from build123d import *

# Parameters (mm, degrees)
SKETCH_1_W               = 17
SKETCH_1_H               = 27
SKETCH_1_R               = 1.5
EXTRUDE_1_DEPTH          = 4
CUT_EXTRUDE_1_DEPTH      = 1
CUT_EXTRUDE_1_DEPTH_BACK = 4
SKETCH_5_W               = 11.75
SKETCH_5_H               = 10
SKETCH_5_R               = 3
EXTRUDE_2_DEPTH          = 4


with BuildPart() as part:
    # Эскиз1 → Бобышка-Вытянуть1 (new body)
    with BuildSketch(Plane.XY):
        with Locations((8.5, 13.5)):
            Rectangle(SKETCH_1_W, SKETCH_1_H)
        with Locations((4, 14.4)):
            Circle(SKETCH_1_R, mode=Mode.SUBTRACT)
        with Locations((4, 4.4)):
            Circle(SKETCH_1_R, mode=Mode.SUBTRACT)
    extrude(amount=EXTRUDE_1_DEPTH)

    # Эскиз2 → Вырез-Вытянуть1 (cut, two sides)
    with BuildSketch(Plane.XY.offset(4)) as cut_extrude_1_sk:
        Polygon((11.25, 5.25), (11.25, 0), (14.25, 0), (14.25, 5.25), (15.5, 5.25), (15.5, 7.75), (14.25, 7.75), (14.25, 13), (11.25, 13), (11.25, 7.75), (10, 7.75), (10, 5.25), align=None)
    extrude(amount=CUT_EXTRUDE_1_DEPTH, mode=Mode.SUBTRACT)
    extrude(cut_extrude_1_sk.sketch, amount=-CUT_EXTRUDE_1_DEPTH_BACK, mode=Mode.SUBTRACT)

    # Эскиз5 → Бобышка-Вытянуть2 (add)
    with BuildSketch(Plane.XY.offset(4)):
        with Locations((-5.875, 22)):
            Rectangle(SKETCH_5_W, SKETCH_5_H)
        with Locations((-6.75, 21.5)):
            Circle(SKETCH_5_R, mode=Mode.SUBTRACT)
    extrude(amount=-EXTRUDE_2_DEPTH)


solid = part.part
The model under review builds one solid part; all positions refer to its coordinate system, in mm. A direction names the side the tool comes from. Round coordinates to 2 decimals unless told otherwise and drop trailing zeros. Loops run counter-clockwise (first coordinate to the right, second up) from the corner with the lowest first, then second, coordinate; pieces in that order, holes last. Notation, with made-up numbers: (80.5, 15.5) -> (88.5, 15.5) arc R32 cw to (88.5, 46.5) -> close; hole circle Ø9 at (-10, 34). An arc over 180 degrees is marked (long way). Answer as CSV lines item,"result".
1) Draft analysis for pull direction Y (two halves, no side actions). For faces 1 (the face through (2, 27, 2)), 2 (the face through (-11.75, 22, 2)), 3 (the face through (-3.98, 20.35, 2.03)), state which applies: pulls with the +Y half, pulls with the -Y half, needs draft (parallel to the pull), parting line crosses it, or undercut.
Geometry results:
face 1,"pulls with the +Y half"
face 2,"needs draft"
face 3,"undercut"
2) Tool access review of faces 4 (the face through (6, 0, 2)), 5 (the face through (14.25, 3, 2)), 6 (the face through (15.5, 6, 2)): name each direction out of +Z, -Z, +X, -X, +Y, -Y from which nothing blocks a thin tool from reaching the whole face with its end or side.
Geometry results:
face 4,"+Z, -Z, +X, -X, -Y"
face 5,"+Z, -Z, -Y"
face 6,"+Z, -Z"
3) For P1, Ø1.2, axis at y = 6.5, z = 2, coming from the -X side, flat-tipped, find the tip position at first contact; note if it passes through.
Geometry results:
P1,"stops at x = 0"
4) To check wall thickness, follow line 1 along X through (y, z) = (9.5, 1.45); line 2 along Y through (x, z) = (14.75, 2.05); line 3 along Y through (x, z) = (-6.75, 1.2). State the ranges of each line that lie inside material, in increasing order. Write a range as from..to.
Geometry results:
line 1,"x = 0..11.25, 14.25..17"
line 2,"y = 0..5.25, 7.75..27"
line 3,"y = 17..18.5, 24.5..27"
5) Add section A-A on x = 4. Write out the cut boundary in (y, z), plus the area to 3 significant figures.
Geometry results:
outline,"(0, 0) -> (2.9, 0) -> (2.9, 4) -> (0, 4) -> close; (5.9, 0) -> (12.9, 0) -> (12.9, 4) -> (5.9, 4) -> close; (15.9, 0) -> (27, 0) -> (27, 4) -> (15.9, 4) -> close"
area,"84.0 mm²"
6) Add section D-D on y = 4.4. Write out the cut boundary in (x, z), plus the area to 3 significant figures.
Geometry results:
outline,"(0, 0) -> (2.5, 0) -> (2.5, 4) -> (0, 4) -> close; (5.5, 0) -> (11.25, 0) -> (11.25, 4) -> (5.5, 4) -> close; (14.25, 0) -> (17, 0) -> (17, 4) -> (14.25, 4) -> close"
area,"44.0 mm²"
7) Add section C-C on z = 1.95. Write out the cut boundary in (x, y).
Geometry results:
outline,"(-11.75, 17) -> (0, 17) -> (0, 0) -> (11.25, 0) -> (11.25, 5.25) -> (10, 5.25) -> (10, 7.75) -> (11.25, 7.75) -> (11.25, 13) -> (14.25, 13) -> (14.25, 7.75) -> (15.5, 7.75) -> (15.5, 5.25) -> (14.25, 5.25) -> (14.25, 0) -> (17, 0) -> (17, 27) -> (-11.75, 27) -> close; hole circle Ø6 at (-6.75, 21.5); hole circle Ø3 at (4, 4.4); hole circle Ø3 at (4, 14.4)"
8) Add section B-B on y = 21.5. Write out the cut boundary in (x, z).
Geometry results:
outline,"(-11.75, 0) -> (-9.75, 0) -> (-9.75, 4) -> (-11.75, 4) -> close; (-3.75, 0) -> (17, 0) -> (17, 4) -> (-3.75, 4) -> close"
